```python
from build123d import *

# Parameters (mm, degrees)
SKETCH1_R           = 1.5
BOSS_EXTRUDE1_DEPTH = 4.5
BOSS_EXTRUDE2_DEPTH = 30
SKETCH3_R           = 1.5
BOSS_EXTRUDE3_DEPTH = 4.5
SKETCH5_R           = 11
BOSS_EXTRUDE4_DEPTH = 2
SKETCH6_R           = 2.5
BOSS_EXTRUDE5_DEPTH = 24
SKETCH7_W           = 14
SKETCH7_H           = 0.5
CUT_EXTRUDE2_DEPTH  = 72.056315694
SKETCH8_W           = 8
SKETCH8_H           = 8.285823085
BOSS_EXTRUDE6_DEPTH = 6.5


with BuildPart() as part:
    # Sketch1 → Boss-Extrude1 (new body)
    with BuildSketch(Plane.XY):
        Polygon((0, 36.5), (5.5, 42), (36.5, 42), (42, 36.5), (42, 5.5), (36.5, 0), (5.5, 0), (0, 5.5), align=None)
        with Locations((5.5, 36.382666597)):
            Circle(SKETCH1_R, mode=Mode.SUBTRACT)
        with Locations((36.5, 36.382666597)):
            Circle(SKETCH1_R, mode=Mode.SUBTRACT)
        with Locations((36.5, 5.382666597)):
            Circle(SKETCH1_R, mode=Mode.SUBTRACT)
        with Locations((5.5, 5.382666597)):
            Circle(SKETCH1_R, mode=Mode.SUBTRACT)
    extrude(amount=BOSS_EXTRUDE1_DEPTH)

    # Sketch2 → Boss-Extrude2 (add)
    with BuildSketch(Plane.XY.offset(4.5)):
        Polygon((8.328427125, 42), (0, 33.671572875), (0, 8.328427125), (8.328427125, 0), (33.671572875, 0), (42, 8.328427125), (42, 33.671572875), (33.671572875, 42), align=None)
    extrude(amount=BOSS_EXTRUDE2_DEPTH)

    # Sketch3 → Boss-Extrude3 (add)
    with BuildSketch(Plane.XY.offset(34.5)):
        Polygon((36.5, 42), (5.5, 42), (0, 36.5), (0, 5.5), (5.5, 0), (36.5, 0), (42, 5.5), (42, 36.5), align=None)
        with Locations((5.5, 5.382666597)):
            Circle(SKETCH3_R, mode=Mode.SUBTRACT)
        with Locations((36.5, 5.382666597)):
            Circle(SKETCH3_R, mode=Mode.SUBTRACT)
        with Locations((5.5, 36.382666597)):
            Circle(SKETCH3_R, mode=Mode.SUBTRACT)
        with Locations((36.5, 36.382666597)):
            Circle(SKETCH3_R, mode=Mode.SUBTRACT)
    extrude(amount=BOSS_EXTRUDE3_DEPTH)

    # Sketch5 → Boss-Extrude4 (add)
    with BuildSketch(Plane(origin=(0, 0, 0), x_dir=(-1, 0, 0), z_dir=(0, 0, -1))):
        with Locations((-21, 21)):
            Circle(SKETCH5_R)
    extrude(amount=BOSS_EXTRUDE4_DEPTH)

    # Sketch6 → Boss-Extrude5 (add)
    with BuildSketch(Plane(origin=(0, 0, -2), x_dir=(-1, 0, 0), z_dir=(0, 0, -1))):
        with Locations((-21, 21)):
            Circle(SKETCH6_R)
    extrude(amount=BOSS_EXTRUDE5_DEPTH)

    # Sketch7 → Cut-Extrude2 (cut, through all)
    with BuildSketch(Plane.ZY):
        with Locations((-19, 23.25)):
            Rectangle(SKETCH7_W, SKETCH7_H)
    extrude(amount=-CUT_EXTRUDE2_DEPTH, mode=Mode.SUBTRACT)

    # Sketch8 → Boss-Extrude6 (add)
    with BuildSketch(Plane.XZ):
        with Locations((17, 32.142911543)):
            Rectangle(SKETCH8_W, SKETCH8_H)
        with Locations((25, 32.142911543)):
            Rectangle(SKETCH8_W, SKETCH8_H)
    extrude(amount=BOSS_EXTRUDE6_DEPTH)


solid = part.part
```
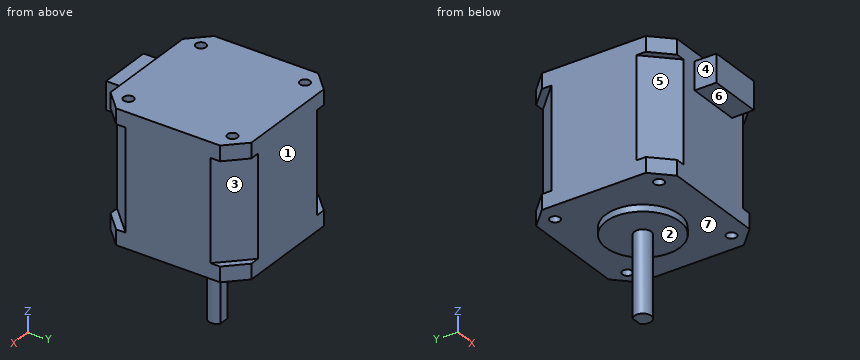
Design review of the part built by this model. Coordinates are the model's own, in mm. Face numbers are marked on the shaded views. A direction names the side the tool comes from. Give positions to 0.01 mm unless a question says otherwise; leave off trailing zeros. Write each loop counter-clockwise with the first axis right and the second up, starting at its lowest first coordinate (ties: lowest second). Pieces come first, ordered by that corner, then holes.
(1) Add section D-D (x = 14.5). Give the boundary of the cut face in (y, z), and give its area (3 significant figures).
Checked values:
outline: (-6.5, 28) - (0, 28) - (0, 0) - (12.13, 0) - (12.13, -2) - (29.87, -2) - (29.87, 0) - (42, 0) - (42, 39) - (0, 39) - (0, 36.29) - (-6.5, 36.29) - close
area: 1,730 mm2
(2) Wall thickness on line 1 along Y through (x, z) = (5.5, 37); line 2 along Z through (x, y) = (5.5, 40.5); line 3 along Z through (x, y) = (14.5, 28): over which ranges is each line inside the solid? List them lowest first.
Checked values:
line 1: y = 0 to 3.88, 6.88 to 34.88, 37.88 to 42
line 2: z = 0 to 4.5, 34.5 to 39
line 3: z = -2 to 39
(3) Clearance check with flat-ended pins moving along their axes: pin 1 Ø2.5 at (x, y) = (5, 5.5) entering from -Z; pin 2 Ø1.8 at (x, y) = (36.5, 36.38) entering from -Z; pin 3 Ø2 at (x, y) = (21, -2.5) entering from +Z. State where each tip first meets the part, or that it passes through.
Checked values:
pin 1: stops at z = 0
pin 2: stops at z = 4.5
pin 3: stops at z = 36.29
(4) Add section B-B (x = 21). Give the boundary of the cut face in (y, z), and give its area (3 significant figures).
Checked values:
outline: (-6.5, 28) - (0, 28) - (0, 0) - (10, 0) - (10, -2) - (18.5, -2) - (18.5, -26) - (23, -26) - (23, -12) - (23.5, -12) - (23.5, -2) - (32, -2) - (32, 0) - (42, 0) - (42, 39) - (0, 39) - (0, 36.29) - (-6.5, 36.29) - close
area: 1,850 mm2
(5) Add section C-C (z = -8.5). Give the boundary of the cut face in (x, y).
Checked values:
outline: circle Ø5 at (21, 21)
(6) Mouldability with a two-part tool opening along Z and no side actions: class the marked faces 1, 2 and 3 as +Z half, -Z half, draft (parallel to the pull), parting line (faces both ways), or undercut.
Checked values:
face 1: draft
face 2: -Z half
face 3: undercut
(7) Add section A-A (y = 21). Give the boundary of the cut face in (x, z), and give its area (3 significant figures).
Checked values:
outline: (0, 0) - (10, 0) - (10, -2) - (18.5, -2) - (18.5, -26) - (23.5, -26) - (23.5, -2) - (32, -2) - (32, 0) - (42, 0) - (42, 39) - (0, 39) - close
area: 1,800 mm2
(8) Tool access review of the marked faces 4, 5, 6 and 7: name each direction out of +Z, -Z, +X, -X, +Y, -Y from which nothing blocks a thin tool from reaching the whole face with its end or side.
Checked values:
face 4: +Z, -Z, -X, -Y
face 5: -X, -Y
face 6: -Z, +X, -X, -Y
face 7: -Z
